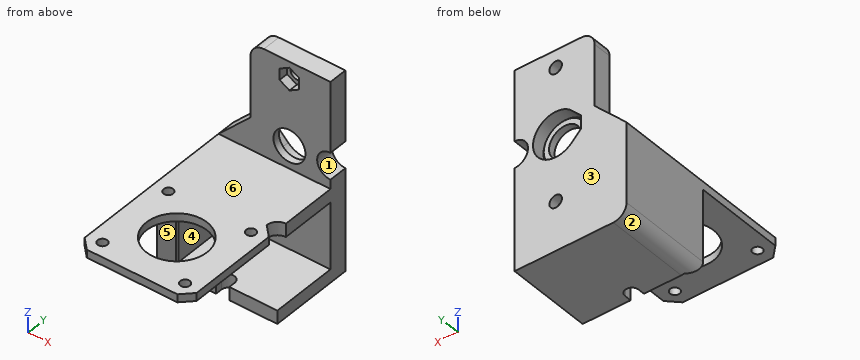
Autodesk Inventor part; units mm, degrees
ref_plane "YZ Plane" through (0, 0, 0) normal (1, 0, 0) x (0, 1, 0)
ref_plane "XZ Plane" through (0, 0, 0) normal (0, 1, 0) x (-1, 0, 0)
ref_plane "XY Plane" through (0, 0, 0) normal (0, 0, 1) x (1, 0, 0)
sketch "Sketch1" plane through (0, 0, 0) normal (0, 1, 0) x (-1, 0, 0)
  line L0 (30, 0) -> (30, -75) construction
  line L1 (30, -75) -> (0, -75) construction
  line L2 (0, -75) -> (0, 0) construction
  line L3 (0, 0) -> (15.4, 0) construction
  line L4 (15.4, 0) -> (15.4, -6.5) construction
  line L5 (15.4, -6.5) -> (0, -6.5) construction
  line L6 (0, -6.5) -> (0, 0) construction
  line L7 (15.4, -6.5) -> (15.4, -31.5) construction
  circle A0 centre (15.4, -31.5) radius 8.5 construction
  line L8 (15.4, -31.5) -> (15.4, -56.5) construction
  circle A1 centre (15.4, -6.5) radius 2.35
  circle A2 centre (15.4, -56.5) radius 2.35
  line L9 (15.4, -23) -> (24.9, -23) construction
  line L10 (24.9, -23) -> (24.9, -40) construction
  line L11 (24.9, -40) -> (15.4, -40) construction
  line L12 (15.4, -40) -> (15.4, -23) construction
  line L13 (5.9, -29) -> (24.9, -29) construction
  line L14 (24.9, -29) -> (24.9, -34) construction
  line L15 (24.9, -34) -> (5.9, -34) construction
  line L16 (5.9, -34) -> (5.9, -29) construction
  line L17 (5.9, -29) -> (24.9, -34) construction
  line L18 (24.9, -29) -> (5.9, -34) construction
  line L19 (24.9, -29) -> (24.9, -34)
  line L20 (24.9, -29) -> (21.4283, -25.5075)
  line L21 (24.9, -34) -> (21.4283, -37.4925)
  arc A3 (21.4283, -25.5075) -> (21.4283, -37.4925) centre (15.4, -31.5) ccw
  arc A4 (0, -36.5) -> (0, -26.5) centre (0, -31.5) ccw
  line L22 (0, 0) -> (0, -26.5)
  line L23 (0, -36.5) -> (0, -75)
  line L24 (42, -40) -> (0, -40) construction
  line L25 (0, -40) -> (0, -75) construction
  line L26 (42, -40) -> (30, -40) construction
  line L27 (30, -40) -> (30, -28) construction
  line L28 (30, -28) -> (42, -28) construction
  line L29 (42, -28) -> (42, -40) construction
  line L30 (30, -28) -> (42, -40)
  line L31 (0, 0) -> (30, 0)
  line L32 (30, -28) -> (30, 0)
  line L33 (42, -40) -> (42, -75)
  line L34 (42, -75) -> (0, -75)
  dimension "d0" = 30
  dimension "d1" = 75
  dimension "d2" = 15.4
  dimension "d3" = 6.5
  dimension "d4" = 25
  dimension "d5" = 17
  dimension "d6" = 25
  dimension "d7" = 4.7
  dimension "d8" = 4.7
  dimension "d9" = 9.5
  dimension "d10" = 5
  dimension "d11" = 5
  dimension "d12" = 42
  dimension "d13" = 35
  dimension "d14" = 12
extrude "Extrusion1" add sketch "Sketch1" against normal blind 7
sketch "Sketch2" plane through (0, -7, 0) normal (0, -1, 0) x (1, 0, 0)
  circle A0 centre (-15.4, -6.5) radius 2.35 construction
  circle A1 centre (-15.4, -56.5) radius 2.35 construction
  line L0 (-15.4, -6.5) -> (-15.4, -10.75) construction
  line L1 (-15.4, -56.5) -> (-15.4, -52.25) construction
  line L2 (-15.4, -10.75) -> (-19.0806, -8.625)
  line L3 (-19.0806, -8.625) -> (-19.0806, -4.375)
  line L4 (-19.0806, -4.375) -> (-15.4, -2.25)
  line L5 (-15.4, -2.25) -> (-11.7194, -4.375)
  line L6 (-11.7194, -4.375) -> (-11.7194, -8.625)
  line L7 (-11.7194, -8.625) -> (-15.4, -10.75)
  line L8 (-15.4, -52.25) -> (-11.7194, -54.375)
  line L9 (-11.7194, -54.375) -> (-11.7194, -58.625)
  line L10 (-11.7194, -58.625) -> (-15.4, -60.75)
  line L11 (-15.4, -60.75) -> (-19.0806, -58.625)
  line L12 (-19.0806, -58.625) -> (-19.0806, -54.375)
  line L13 (-19.0806, -54.375) -> (-15.4, -52.25)
  point P0 (0, 0)
  dimension "d18" = 4.25
  dimension "d19" = 4.25
extrude "Extrusion2" cut sketch "Sketch2" against normal blind 3.5
sketch "Sketch3" plane through (0, -7, 0) normal (0, -1, 0) x (1, 0, 0)
  arc A0 (-21.4283, -37.4925) -> (-21.4283, -25.5075) centre (-15.4, -31.5) ccw
  circle A1 centre (-15.4, -31.5) radius 6
  line L0 (-24.9, -29) -> (-21.4283, -25.5075)
  line L1 (-24.9, -34) -> (-24.9, -29)
  line L2 (-21.4283, -37.4925) -> (-24.9, -34)
  point P0 (0, 0)
  dimension "d22" = 12
extrude "Extrusion3" add sketch "Sketch3" against normal blind 2.1
sketch "Sketch4" plane through (0, -4.9, 0) normal (0, 1, 0) x (1, 0, 0)
  circle A0 centre (-15.4, 31.5) radius 6
  circle A1 centre (-15.4, 31.5) radius 8
  point P0 (0, 0)
  dimension "d25" = 16
extrude "Extrusion4" add sketch "Sketch4" along normal blind 0.5
sketch "Sketch5" plane through (0, -7, 0) normal (0, -1, 0) x (1, 0, 0)
  line L0 (0, -75) -> (0, -36.5) construction
  line L1 (-42, -70) -> (-42, -40) construction
  line L2 (0, -75) -> (-42, -75) construction
  line L3 (-42, -75) -> (-42, -40) construction
  line L4 (-42, -40) -> (0, -40) construction
  line L5 (0, -40) -> (0, -75) construction
  line L6 (0, -40) -> (-42, -40) construction
  line L7 (-42, -40) -> (-42, -45) construction
  line L8 (-42, -45) -> (0, -45) construction
  line L9 (0, -45) -> (0, -40) construction
  line L10 (-42, -40) -> (-37, -40) construction
  line L11 (-37, -40) -> (-37, -75) construction
  line L12 (-37, -75) -> (-42, -75) construction
  line L13 (-42, -75) -> (-42, -40) construction
  line L14 (-42, -75) -> (0, -75) construction
  line L15 (0, -75) -> (0, -70) construction
  line L16 (0, -70) -> (-42, -70) construction
  line L17 (-42, -70) -> (-42, -75) construction
  line L18 (-37, -75) -> (0, -75)
  line L19 (0, -75) -> (0, -70)
  line L20 (-37, -70) -> (0, -70)
  line L21 (-37, -45) -> (-37, -70)
  line L22 (0, -40) -> (-42, -40)
  line L23 (0, -45) -> (0, -40)
  line L24 (-37, -45) -> (0, -45)
  line L25 (-42, -40) -> (-42, -75)
  line L26 (-42, -40) -> (-42, -75)
  line L27 (-42, -75) -> (0, -75)
  point P0 (0, 0)
  dimension "d28" = 5
  dimension "d29" = 5
extrude "Extrusion5" add sketch "Sketch5" along normal blind 25
sketch "Sketch6" plane through (-42, -7, -40) normal (0, 0, 1) x (1, 0, 0)
  line L0 (5, -25) -> (42, -25)
  line L1 (38, -25) -> (0, -25)
  line L2 (0, -25) -> (0, -63)
  line L3 (4, -67) -> (38, -67)
  line L4 (42, -63) -> (42, -29)
  line L5 (42, -63) -> (38, -67)
  line L6 (4, -67) -> (0, -63)
  line L7 (42, -29) -> (38, -25)
  circle A0 centre (21, -46) radius 11.4
  line L8 (36.5, -61.5) -> (5.5, -61.5) construction
  line L9 (5.5, -61.5) -> (5.5, -30.5) construction
  line L10 (5.5, -30.5) -> (36.5, -30.5) construction
  line L11 (36.5, -30.5) -> (36.5, -61.5) construction
  line L12 (36.5, -61.5) -> (5.5, -30.5) construction
  line L13 (5.5, -61.5) -> (36.5, -30.5) construction
  circle A1 centre (36.5, -61.5) radius 1.8
  circle A2 centre (5.5, -61.5) radius 1.8
  circle A3 centre (5.5, -30.5) radius 1.8
  circle A4 centre (36.5, -30.5) radius 1.8
  point P0 (42, 7)
  point P1 (0, -67)
  point P2 (42, -67)
  dimension "d32" = 42
  dimension "d33" = 42
  dimension "d34" = 4
  dimension "d35" = 4
  dimension "d36" = 4
  dimension "d37" = 4
  dimension "d38" = 4
  dimension "d39" = 4
  dimension "d40" = 22.8
  dimension "d41" = 31
  dimension "d42" = 31
  dimension "d43" = 3.6
  dimension "d44" = 3.6
  dimension "d45" = 3.6
  dimension "d46" = 3.6
extrude "Extrusion6" add sketch "Sketch6" against normal blind 3
sketch "Sketch7" plane through (-42, -7, -40) normal (0, 0, 1) x (1, 0, 0)
  line L0 (42, -25) -> (38, -25)
  arc A0 (42, -21) -> (38, -25) centre (42, -25) ccw
  line L1 (42, -21) -> (42, -25)
  point P0 (42, 7)
extrude "Extrusion7" cut sketch "Sketch7" against normal blind 5
sketch "Sketch8" plane through (0, 0, -75) normal (0, 0, -1) x (-1, 0, 0)
  line L0 (42, -32) -> (0, -32) construction
  line L1 (20.5, -34.5) -> (20.5, -29.5) construction
  line L2 (37, -32) -> (4, -32) construction
  line L3 (23, -34.5) -> (23, -29.5) construction
  line L4 (18, -29.5) -> (18, -34.5) construction
  arc A0 (18, -34.5) -> (23, -34.5) centre (20.5, -34.5) ccw construction
  arc A1 (23, -29.5) -> (18, -29.5) centre (20.5, -29.5) ccw construction
  line L5 (20.5, -32) -> (25.5, -32) construction
  arc A2 (23, -29.5) -> (18, -29.5) centre (20.5, -29.5) ccw
  line L6 (23, -29.5) -> (23, -32)
  line L7 (18, -29.5) -> (18, -32)
  line L8 (18, -32) -> (23, -32)
  point P0 (0, 0)
  dimension "d51" = 2.5
  dimension "d52" = 90
  dimension "d53" = 5
extrude "Extrusion8" cut sketch "Sketch8" against normal blind 5
sketch "Sketch9" plane through (-42, -7, -43) normal (0, 0, -1) x (-1, 0, 0)
  line L0 (0, -25) -> (-19, -25) construction
  line L1 (0, -25) -> (-4, -25) construction
  line L2 (-4, -25) -> (-4, -29) construction
  line L3 (-4, -29) -> (0, -29) construction
  line L4 (0, -29) -> (0, -25) construction
  line L5 (0, -29) -> (-4, -25)
  line L6 (0, -25) -> (-4, -25)
  line L7 (0, -25) -> (0, -29)
  line L8 (0, 0) -> (0, -63)
  point P0 (-42, 7)
  dimension "d56" = 4
  dimension "d57" = 4
extrude "Extrusion9" add sketch "Sketch9" along normal up to surface (32 mm away)
fillet "Fillet1" radius 5 2 edges at (-30, -3.5, 0) (-42, -18, -75)
equation "\"d38\" = d34"
equation "\"d39\" = d38"
Check sheet for the modelled part. Datum: model origin and axes. Units: mm. Face numbers are marked on the shaded views. A direction names the side the tool comes from. Round coordinates to 2 decimals unless told otherwise and drop trailing zeros. Loops run counter-clockwise (first coordinate to the right, second up) from the corner with the lowest first, then second, coordinate; pieces in that order, holes last. Notation, with made-up numbers: (30.25, -7.75) - (60.25, -7.75) arc R22 cw to (60.25, -0.75) - close; hole circle Ø2 at (1.25, 17.5). An arc over 180 degrees is marked (long way). Write item = value, one per line. Start each with the question number.
Q1. Section check B-B (z = -6.5). Record the boundary of the cut face in (x, y).
Q2. Section check D-D (z = -63). Record the boundary of the cut face in (x, y), plus the area to 3 significant figures.
Q3. Depth check by flat-ended pin: P1, Ø4, axis at x = -5.5, y = -68.5, coming from the +Z side; P2, Ø5.5, axis at y = -5, z = -13, coming from the -X side; P3, Ø8, axis at x = -22, z = -54.5, coming from the -Y side; P4, Ø11, axis at x = -15.4, z = -31.5, coming from the -Y side. Enter the tip coordinate at first touch or a pass-through.
Q4. Section check C-C (x = -31). Record the boundary of the cut face in (y, z), plus the area to 3 significant figures.
Q5. Access from +Z, -Z, +X, -X, +Y, -Y to the whole of each face (thin tool, end or side, straight path). Record for the marked faces 4, 5 and 6.
Q6. Release check for a two-part mould opening along Z. For the marked faces 1, 2 and 3 record: pulls with the +Z half, pulls with the -Z half, needs draft (parallel to the pull), parting line crosses it, or undercut.
Q7. Section check A-A (y = -68.5). Record the boundary of the cut face in (x, z), plus the area to 3 significant figures.
Q8. Thickness scan on L1, parallel to Y at x = -36.5, z = -40.75; L2, parallel to Z at x = -15.4, y = -2.35; L3, parallel to Z at x = -34, y = -15. Record the ranges inside material, lowest first.
Derived:
q1.outline = (-30, -7) - (-19.08, -7) - (-19.08, -3.5) - (-17.75, -3.5) - (-17.75, 0) - (-30, 0) - close; (-13.05, -3.5) - (-11.72, -3.5) - (-11.72, -7) - (0, -7) - (0, 0) - (-13.05, 0) - close
q2.outline = (-42, -36) - (-38, -32) - (-37, -32) - (-37, -7) - (0, -7) - (0, 0) - (-42, 0) - close
q2.area = 427 mm^2
q3.P1 = -40
q3.P2 = -30
q3.P3 = -7
q3.P4 = through
q4.outline = (-74, -43) - (-58.47, -43) - (-58.47, -40) - (-74, -40) - close; (-47.53, -43) - (-32, -43) - (-32, -45) - (-7, -45) - (-7, -70) - (-32, -70) - (-32, -75) - (0, -75) - (0, -29) - (-7, -29) - (-7, -40) - (-47.53, -40) - close
q4.area = 665 mm^2
q5.face_4 = +X, -Y
q5.face_5 = -Z, +X, -Y
q5.face_6 = +Z, +X, -X, -Y
q6.face_1 = undercut
q6.face_2 = pulls with the -Z half
q6.face_3 = needs draft
q7.outline = (-42, -43) - (-38.3, -43) - (-38.3, -40) - (-42, -40) - close; (-34.7, -43) - (-7.3, -43) - (-7.3, -40) - (-34.7, -40) - close; (-3.7, -43) - (0, -43) - (0, -40) - (-3.7, -40) - close
q7.area = 104 mm^2
q8.L1 = -74 to -70.3, -66.7 to -39.3, -35.7 to 0
q8.L2 = -75 to -58.85, -54.15 to -40, -23 to -8.85, -4.15 to 0
q8.L3 = -75 to -70, -45 to -40
